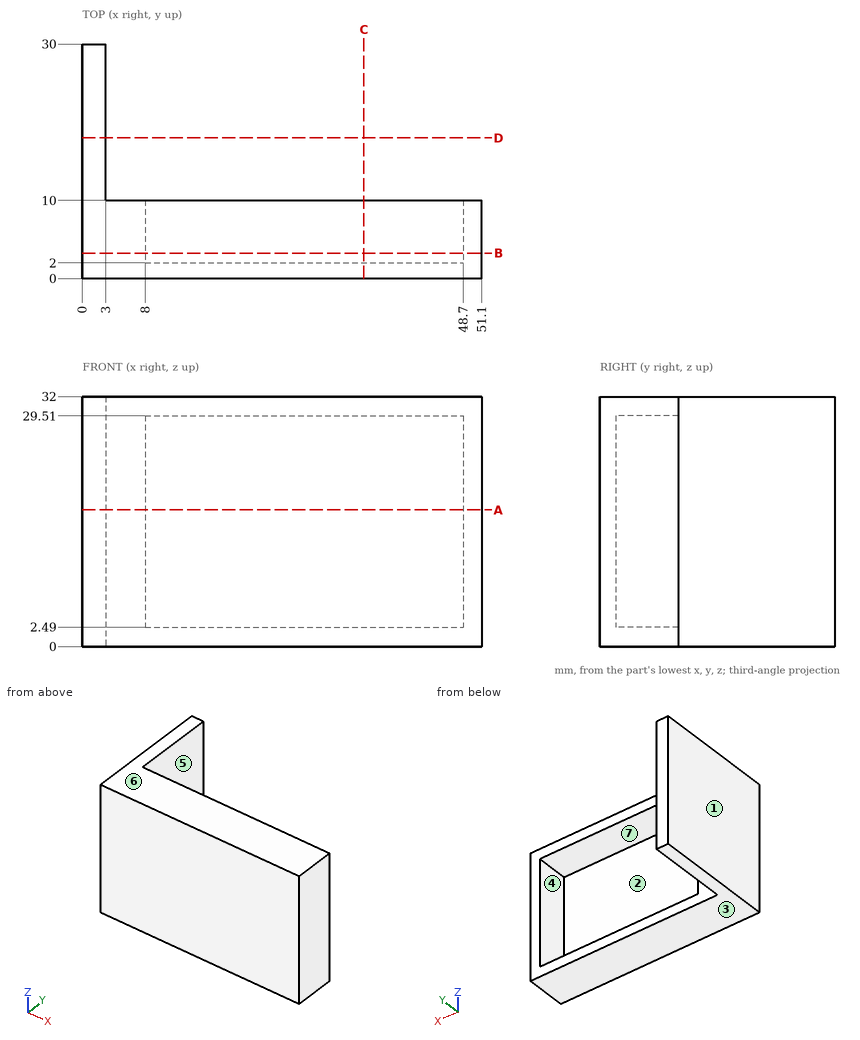
Answer from the drawing. Dimensions are ordinates in mm from the lowest x, y and z of the part. A direction names the side the tool comes from. Coordinates: 2 decimals unless noted, no trailing zeros. Write each loop counter-clockwise with the first axis right and the second up, starting at its lowest first coordinate (ties: lowest second). Pieces come first, ordered by that corner, then holes. Notation, with made-up numbers: (-27.75, -16) -> (14.25, -16) arc R22 cw to (14.25, 21) -> close; hole circle Ø5 at (30.5, 49.5). An arc over 180 degrees is marked (long way). One line per question, with ' | ' between items.
1. Section B-B (y = 3.25) is taken. Determine the outline of the cut face in (x, z).
Verdict:
outline: (0, 0) -> (51.1, 0) -> (51.1, 32) -> (0, 32) -> close; hole (8, 2.49) -> (48.7, 2.49) -> (48.7, 29.51) -> (8, 29.51) -> close
2. Section D-D (y = 18) is taken. Determine the outline of the cut face in (x, z).
Verdict:
outline: (0, 0) -> (3, 0) -> (3, 32) -> (0, 32) -> close
3. Section A-A (z = 17.5) is taken. Determine the outline of the cut face in (x, y).
Verdict:
outline: (0, 0) -> (51.1, 0) -> (51.1, 10) -> (48.7, 10) -> (48.7, 2) -> (8, 2) -> (8, 10) -> (3, 10) -> (3, 30) -> (0, 30) -> close
4. For a pull along X with two mould halves and no side action, classify the marked faces 1, 2, 3 and 4 as released by +X, released by -X, zero draft, split by the parting line, or undercut.
Verdict:
face 1: released by -X | face 2: undercut | face 3: zero draft | face 4: undercut
5. Given pin 1 Ø8 at (x, y) = (42, 14.5) entering from +Z; pin 2 Ø3 at (y, z) = (12, 8) entering from +X; pin 3 Ø12 at (x, z) = (12, 14) entering from +Y; pin 4 Ø16 at (x, z) = (27, 13.5) entering from +Y, each flat-ended and moving along its own axis, determine where each tip first touches the part or whether it passes through.
Verdict:
pin 1: passes through | pin 2: stops at x = 3 | pin 3: stops at y = 10 | pin 4: stops at y = 2
6. Straight lines are drawn through the part: line 1 (X direction, y = 9.5, z = 5); line 2 (Z direction, x = 15.5, y = 7.75); line 3 (Y direction, x = 39, z = 11). For each, find the intervals that lie inside material, in ascending order.
Verdict:
line 1: x = 0 to 8, 48.7 to 51.1 | line 2: z = 0 to 2.49, 29.51 to 32 | line 3: y = 0 to 2
7. Which of the six approach directions +Z, -Z, +X, -X, +Y, -Y give full straight-line access (tool end or side, diameter ignored) to the marked faces 5, 6 and 7?
Verdict:
face 5: +Z, -Z, +X, +Y | face 6: +Z, +X, -X, +Y, -Y | face 7: +Y
8. Section C-C (x = 36) is taken. Determine the outline of the cut face in (y, z).
Verdict:
outline: (0, 0) -> (10, 0) -> (10, 2.49) -> (2, 2.49) -> (2, 29.51) -> (10, 29.51) -> (10, 32) -> (0, 32) -> close
